For this review, use the dimensioned drawing (mm, ordinates from the lowest corner) and the shaded views. Coordinates: 2 decimals unless noted, no trailing zeros. Order: outer loops, then holes, each group sorted by start corner. A loop starts at its lowest first (then second) coordinate and runs counter-clockwise, first axis right, second up. Notation, with made-up numbers: M 24,-16 L 30,-16 A36 cw 30,23 Z; hole C 41.25,62.5 d11. An arc over 180 degrees is marked long. Use CSV: the item, a comma, the result in double quotes.
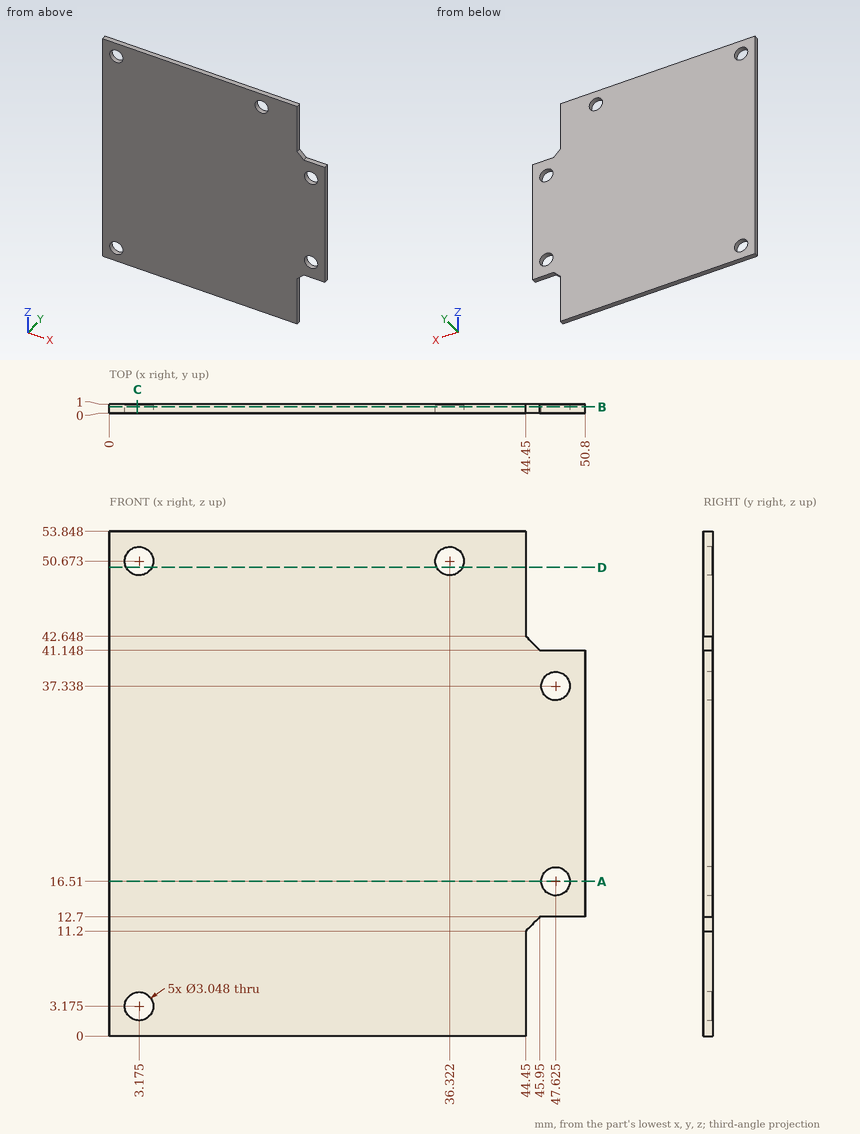
Item 1: Add section C-C on x = 3. State the section outline as (y, z) points.
Solutions:
outline,"M 0,0 L 1,0 L 1,1.66 L 0,1.66 Z; M 0,4.69 L 1,4.69 L 1,49.16 L 0,49.16 Z; M 0,52.19 L 1,52.19 L 1,53.85 L 0,53.85 Z"
Item 2: Add section A-A on z = 16.51. State the section outline as (x, y) points.
Solutions:
outline,"M 0,0 L 46.1,0 L 46.1,1 L 0,1 Z; M 49.15,0 L 50.8,0 L 50.8,1 L 49.15,1 Z"
Item 3: Clearance check with flat-ended pins moving along their axes: pin 1 Ø0.5 at (y, z) = (0.5, 46) entering from +X; pin 2 Ø0.5 at (x, y) = (47.5, 0.5) entering from +Z. State where each tip first meets the part, or that it passes through.
Solutions:
pin 1,"x = 44.45"
pin 2,"z = 41.15"
Item 4: Add section D-D on z = 50. State the section outline as (x, y) points, and give its area (3 significant figures).
Solutions:
outline,"M 0,0 L 1.81,0 L 1.81,1 L 0,1 Z; M 4.54,0 L 34.95,0 L 34.95,1 L 4.54,1 Z; M 37.69,0 L 44.45,0 L 44.45,1 L 37.69,1 Z"
area,"39.0 mm^2"
Item 5: To check wall thickness, follow line 1 along X through (y, z) = (0.65, 37.5); line 2 along X through (y, z) = (0.25, 44.5); line 3 along Z through (x, y) = (35.5, 0.15). State the ranges of each line that lie inside material, in increasing order. Write a range as [from, to].
Solutions:
line 1,"[0, 46.11], [49.14, 50.8]"
line 2,"[0, 44.45]"
line 3,"[0, 49.39], [51.96, 53.85]"
Item 6: Add section B-B on y = 0.7. State the section outline as (x, z) points (3 decimals).
Solutions:
outline,"M 0,0 L 44.45,0 L 44.45,11.2 L 45.95,12.7 L 50.8,12.7 L 50.8,41.148 L 45.95,41.148 L 44.45,42.648 L 44.45,53.848 L 0,53.848 Z; hole C 3.175,3.175 d3.048; hole C 3.175,50.673 d3.048; hole C 36.322,50.673 d3.048; hole C 47.625,16.51 d3.048; hole C 47.625,37.338 d3.048"
